```python
from build123d import *

# Parameters (mm, degrees)
SKETCH1_R           = 1.4224
BOSS_EXTRUDE1_DEPTH = 2.54
SKETCH2_R           = 2.286
SKETCH2_R_2         = 3.175
CUT_EXTRUDE1_DEPTH  = 3.54


with BuildPart() as part:
    # Sketch1 → Boss-Extrude1 (new body)
    with BuildSketch(Plane(origin=(0, 0, 0), x_dir=(1, 0, 0), z_dir=(0, 1, 0))):
        with BuildLine():
            Line((-73.66, 76.2), (73.66, 76.2))
            ThreePointArc((73.66, 76.2), (75.456051224, 75.456051224), (76.2, 73.66))
            Line((76.2, 73.66), (76.2, -73.66))
            ThreePointArc((76.2, -73.66), (75.456051224, -75.456051224), (73.66, -76.2))
            Line((73.66, -76.2), (-73.66, -76.2))
            ThreePointArc((-73.66, -76.2), (-75.456051224, -75.456051224), (-76.2, -73.66))
            Line((-76.2, -73.66), (-76.2, 73.66))
            ThreePointArc((-76.2, 73.66), (-75.456051224, 75.456051224), (-73.66, 76.2))
        make_face()
        Circle(SKETCH1_R, mode=Mode.SUBTRACT)
    extrude(amount=BOSS_EXTRUDE1_DEPTH)

    # Sketch2 → Cut-Extrude1 (cut, through all)
    with BuildSketch(Plane(origin=(0, 2.54, 0), x_dir=(1, 0, 0), z_dir=(0, 1, 0))):
        with Locations((-38.1, 51.05145896)):
            Circle(SKETCH2_R)
        with Locations((38.1, 51.05145896)):
            Circle(SKETCH2_R)
        with Locations((38.1, -52.221692976)):
            Circle(SKETCH2_R)
        with Locations((-38.1, -52.221692976)):
            Circle(SKETCH2_R)
        Circle(SKETCH2_R_2)
    extrude(amount=-CUT_EXTRUDE1_DEPTH, mode=Mode.SUBTRACT)


solid = part.part
```
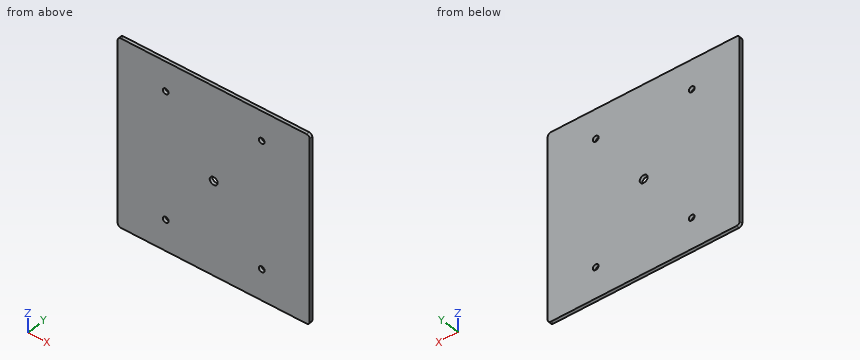
Verification items for the finished model (mm, model axes). Give positions to 0.01 mm unless a question says otherwise; leave off trailing zeros. Loops run counter-clockwise (first coordinate to the right, second up) from the corner with the lowest first, then second, coordinate; pieces in that order, holes last.
1. Section check B-B, the plane x = -38.1. Enter the section's corners in (y, z), then the cut area to 3 significant figures.
2. Section check A-A, the plane x = 0. Enter the section's corners in (y, z) (3 decimals).
3. Thickness scan on line 1 (Z direction, x = 38.1, y = 0.7); line 2 (X direction, y = 0.45, z = -49); line 3 (X direction, y = 1.45, z = -52). Record the ranges inside material, lowest first.
4. Go/stop test with a flat-tipped pin: pin 1 Ø3.5 at (x, z) = (38.1, -51.05) entering from +Y. Record where the tip stops, or that it passes through.
Geometry says:
1. outline: (0, -76.2) - (2.54, -76.2) - (2.54, -53.34) - (0, -53.34) - close; (0, -48.77) - (2.54, -48.77) - (2.54, 49.94) - (0, 49.94) - close; (0, 54.51) - (2.54, 54.51) - (2.54, 76.2) - (0, 76.2) - close
1. area: 364 mm2
2. outline: (0, -76.2) - (2.54, -76.2) - (2.54, -3.175) - (0, -3.175) - close; (0, 3.175) - (2.54, 3.175) - (2.54, 76.2) - (0, 76.2) - close
3. line 1: z = -76.2 to -53.34, -48.77 to 49.94, 54.51 to 76.2
3. line 2: x = -76.2 to -39.11, -37.09 to 37.09, 39.11 to 76.2
3. line 3: x = -76.2 to -40.18, -36.02 to 36.02, 40.18 to 76.2
4. pin 1: passes through
